```python
from build123d import *

# Parameters (mm, degrees)
F0_R     = 10.9982
F1_DEPTH = 8.89


with BuildPart() as f1:
    # F0 (on Top) → F1 (new body)
    with BuildSketch(Plane.XY):
        with BuildLine():
            ThreePointArc((-7.30594, -20.586929), (-7.114139, -19.208105), (-7.050024, -17.817482))
            ThreePointArc((-7.050024, -17.817482), (-12.08059, -6.559271), (-23.823306, -2.795956))
            ThreePointArc((-23.823306, -2.795956), (-33.238608, -28.100195), (-7.30594, -20.586929))
        make_face()
        with Locations((-22.163024, -17.817482)):
            Circle(F0_R, mode=Mode.SUBTRACT)
        with BuildLine():
            ThreePointArc((-23.823306, -2.795956), (-12.08059, -6.559271), (-7.050024, -17.817482))
            ThreePointArc((-7.050024, -17.817482), (-7.114139, -19.208105), (-7.30594, -20.586929))
            ThreePointArc((-7.30594, -20.586929), (0.735892, -19.274873), (8.464534, -21.855699))
            ThreePointArc((8.464534, -21.855699), (10.732709, -8.182627), (23.190467, -2.107943))
            ThreePointArc((23.190467, -2.107943), (16.953024, 11.468692), (15.070929, 26.290583))
            ThreePointArc((15.070929, 26.290583), (0.05546, 12.304565), (-15.062253, 26.180002))
            ThreePointArc((-15.062253, 26.180002), (-17.092318, 10.981347), (-23.823306, -2.795956))
        make_face()
        Circle(F0_R, mode=Mode.SUBTRACT)
        with BuildLine():
            ThreePointArc((-15.113, 27.417463), (-15.083625, 26.798897), (-15.062253, 26.180002))
            ThreePointArc((-15.062253, 26.180002), (0.05546, 12.304565), (15.070929, 26.290583))
            ThreePointArc((15.070929, 26.290583), (15.088741, 26.854143), (15.113, 27.417463))
            ThreePointArc((15.113, 27.417463), (0, 42.530463), (-15.113, 27.417463))
        make_face()
        with Locations((0, 27.417463)):
            Circle(F0_R, mode=Mode.SUBTRACT)
        with BuildLine():
            ThreePointArc((-15.113, 27.417463), (-15.100308, 26.798212), (-15.062253, 26.180002))
            ThreePointArc((-15.062253, 26.180002), (-15.083625, 26.798897), (-15.113, 27.417463))
        make_face()
        with BuildLine():
            ThreePointArc((23.190467, -2.107943), (10.732709, -8.182627), (8.464534, -21.855699))
            ThreePointArc((8.464534, -21.855699), (25.195882, -32.146581), (37.96106, -17.217064))
            ThreePointArc((37.96106, -17.217064), (33.654946, -6.652312), (23.190467, -2.107943))
        make_face()
        with Locations((22.84806, -17.217064)):
            Circle(F0_R, mode=Mode.SUBTRACT)
        with BuildLine():
            ThreePointArc((15.113, 27.417463), (15.088741, 26.854143), (15.070929, 26.290583))
            ThreePointArc((15.070929, 26.290583), (15.102479, 26.85363), (15.113, 27.417463))
        make_face()
    extrude(amount=F1_DEPTH)


solid = f1.part
```
For this review, take the finished solid that the model builds, in its own axes (mm). Round coordinates to 2 decimals unless told otherwise and drop trailing zeros. Write each loop counter-clockwise with the first axis right and the second up, starting at its lowest first coordinate (ties: lowest second). Pieces come first, ordered by that corner, then holes. Notation, with made-up numbers: M 87.25,63 L 103.25,63 A26 cw 103.25,80 Z; hole C 50,47 d5. An arc over 180 degrees is marked long. One line per item, written item: value. Start each with the question number.
(1) The part is to be moulded in two halves that separate along Y. For faces 1 (the cylindrical face through (-8.73, -6.69, 4.38)), 2 (the cylindrical face through (0.332, 42.527, 4.383)), 3 (the cylindrical face through (0.621, -19.266, 4.383)), say which applies: released by +Y, released by -Y, zero draft, split by the parting line, or undercut.
(2) We need section A-A (y = 0). Give the boundary of the cut face in (x, z), and give its area (3 significant figures).
(3) Wall thickness on line 1 (Y direction, x = 0, z = 2.75); line 2 (Y direction, x = 6, z = 1); line 3 (X direction, y = -8, z = 7.75): over which ranges is each line inside the solid? List them lowest first.
(4) We need section B-B (x = 0). Give the boundary of the cut face in (y, z).
(5) Insertion check: pin 1 (2 mm diameter, centred on y = 27.5, z = 6.5, fed in from +X); pin 2 (3 mm diameter, centred on x = 15, y = -6.5, fed in from -Z). Each pin has a flat end and moves straight along its axis. Give the tip position at first contact, or say it passes through.
(6) We need section C-C (z = 5.5). Give the boundary of the cut face in (x, y), and give its area (3 significant figures).
(7) We need section D-D (x = -31.5). Give the boundary of the cut face in (y, z), and give its area (3 significant figures).
Result:
1. face 1: undercut
1. face 2: released by +Y
1. face 3: released by -Y
2. outline: M -21.99,0 L -11,0 L -11,8.89 L -21.99,8.89 Z; M 11,0 L 21.88,0 L 21.88,8.89 L 11,8.89 Z
2. area: 194 mm²
3. line 1: -19.23 to -11, 11 to 16.42, 38.42 to 42.53
3. line 2: -20.57 to -9.22, 9.22 to 18.2, 36.63 to 41.29
3. line 3: -33.65 to -27.12, -17.21 to -7.55, 7.55 to 16.85, 28.85 to 34.83
4. outline: M -19.23,0 L -11,0 L -11,8.89 L -19.23,8.89 Z; M 11,0 L 16.42,0 L 16.42,8.89 L 11,8.89 Z; M 38.42,0 L 42.53,0 L 42.53,8.89 L 38.42,8.89 Z
5. pin 1: x = 15.11
5. pin 2: z = 0
6. outline: M -23.82,-2.8 A15.11 ccw long -7.31,-20.59 A17 cw 8.46,-21.86 A15.11 ccw long 23.19,-2.11 A49.28 cw 15.07,26.29 A15.11 ccw 15.11,27.42 A15.11 ccw -15.11,27.42 A15.11 ccw -15.06,26.18 A47.88 cw Z; hole C -22.16,-17.82 d22; hole C 0,0 d22; hole C 0,27.42 d22; hole C 22.85,-17.22 d22
6. area: 1,680 mm²
7. outline: M -29.7,0 L -23.63,0 L -23.63,8.89 L -29.7,8.89 Z; M -12.01,0 L -5.93,0 L -5.93,8.89 L -12.01,8.89 Z
7. area: 108 mm²
